```python
from build123d import *

# Parameters (mm, degrees)
EXTRUDE_1_DEPTH        = 3
SKETCH_2_R             = 4
EXTRUDE_2_DEPTH        = 10
PATTERN_LINEAR_1_COUNT = 3
PATTERN_LINEAR_1_PITCH = 20
SKETCH_3_R             = 1.5
CUT_EXTRUDE_1_DEPTH    = 65
SKETCH_4_R             = 2.5
CUT_EXTRUDE_2_DEPTH    = 66.192024052


with BuildPart() as part:
    # 草图1 → 凸台-拉伸1 (new body)
    with BuildSketch(Plane(origin=(0, 0, 0), x_dir=(1, 0, 0), z_dir=(0, 1, 0))):
        Polygon((0, 25), (60, 25), (60, -25), (0, -25), (0, -15), (5, -15), (5, -5), (0, -5), (0, 5), (5, 5), (5, 15), (0, 15), align=None)
    extrude(amount=EXTRUDE_1_DEPTH)

    # 草图2 → 凸台-拉伸2 (add)
    with BuildSketch(Plane.XY.offset(-25)):
        with Locations((0, 4)):
            Circle(SKETCH_2_R)
    extrude_2 = extrude(amount=EXTRUDE_2_DEPTH)

    # 阵列(线性)1: 凸台-拉伸2 ×3
    with Locations(*[(0, 0, i * PATTERN_LINEAR_1_PITCH) for i in range(1, PATTERN_LINEAR_1_COUNT)]):
        add(extrude_2)

    # 草图3 → 切除-拉伸1 (cut, symmetric)
    with BuildSketch(Plane.XY.offset(-25)):
        with Locations((0, 4)):
            Circle(SKETCH_3_R)
    extrude(amount=CUT_EXTRUDE_1_DEPTH, both=True, mode=Mode.SUBTRACT)

    # 草图4 → 切除-拉伸2 (cut, through all)
    with BuildSketch(Plane(origin=(0, 3, 0), x_dir=(1, 0, 0), z_dir=(0, 1, 0))):
        with Locations(Location((40, 15, 0), (0, 0, 270))):
            Circle(SKETCH_4_R)
        with Locations(Location((40, 0, 0), (0, 0, 270))):
            Circle(SKETCH_4_R)
        with Locations(Location((40, -15, 0), (0, 0, 270))):
            Circle(SKETCH_4_R)
    extrude(amount=-CUT_EXTRUDE_2_DEPTH, mode=Mode.SUBTRACT)

    # 草图10 → 切除-旋转1 (revolve, cut)
    with BuildSketch(Plane(origin=(40, 0, 0), x_dir=(0, 0, -1), z_dir=(1, 0, 0))):
        Polygon((12.5, 3), (10.5, 3), (12.5, 1), align=None)
    revolve(axis=Axis((40, 0, -15), (0, 1, 0)), mode=Mode.SUBTRACT)

    # 草图11 → 切除-旋转2 (revolve, cut)
    with BuildSketch(Plane(origin=(40, 0, 0), x_dir=(0, 0, -1), z_dir=(1, 0, 0))):
        Polygon((-2.5, 3), (-4.5, 3), (-2.5, 1), align=None)
    revolve(axis=Axis((40, 0, 0), (0, 1, 0)), mode=Mode.SUBTRACT)

    # 草图12 → 切除-旋转3 (revolve, cut)
    with BuildSketch(Plane(origin=(40, 0, 0), x_dir=(0, 0, -1), z_dir=(1, 0, 0))):
        Polygon((-17.5, 3), (-19.5, 3), (-17.5, 1), align=None)
    revolve(axis=Axis((40, 0, 15), (0, 1, 0)), mode=Mode.SUBTRACT)


solid = part.part
```
For this review, take the finished solid that the model builds, in its own axes (mm). A direction names the side the tool comes from. Coordinates: 2 decimals unless noted, no trailing zeros. Write each loop counter-clockwise with the first axis right and the second up, starting at its lowest first coordinate (ties: lowest second). Pieces come first, ordered by that corner, then holes.
(1) For pin 1 Ø1 at (x, z) = (53, -6) entering from +Y; pin 2 Ø2.5 at (x, y) = (0, 4) entering from +Z; pin 3 Ø2.5 at (y, z) = (1, -10) entering from -X; pin 4 Ø8 at (x, z) = (40, 15) entering from +Y, all flat-tipped, find the tip position at first contact; note any pin that passes through.
(2) Wall thickness on probe 1 along Y at (x, z) = (0, -21); probe 2 along Y at (x, z) = (31, -11.5); probe 3 along X at (y, z) = (1.25, -17): over which ranges is each line inside the solid? List them lowest first.
(3) Add section A-A on x = 40. Give the boundary of the cut face in (y, z).
(4) Add section C-C on z = 6.5. Give the boundary of the cut face in (x, y), then the cut area to 3 significant figures.
(5) Tool access review of faces 5 (the face through (0.806, 5.265, -19.93)), 6 (the face through (1.44, 3.17, -15)): name each direction out of +Z, -Z, +X, -X, +Y, -Y from which nothing blocks a thin tool from reaching the whole face with its end or side.
(6) Add section D-D on x = 32. Give the boundary of the cut face in (y, z), then the cut area to 3 significant figures.
(7) The part is to be moulded in two halves that separate along X. For faces 1 (the face through (5, 1, 10)), 2 (the face through (30, 0, 0)), 3 (the face through (37.56, 0.51, 14.46)), 4 (the face through (60, 1, 0)), say which applies: +X half, -X half, draft (parallel to the pull), parting line (faces both ways), or undercut.
(8) Add section B-B on y = 4. Give the boundary of the cut face in (x, z), then the cut area to 3 significant figures.
Answer sheet:
1. pin 1: stops at y = 3
1. pin 2: passes through
1. pin 3: stops at x = 5
1. pin 4: stops at y = 2.5
2. probe 1: y = 0 to 2.5, 5.5 to 8
2. probe 2: y = 0 to 3
2. probe 3: x = -2.9 to 38.11, 41.89 to 60
3. outline: (0, -25) - (3, -25) - (3, -19.5) - (1, -17.5) - (0, -17.5) - close; (0, -12.5) - (1, -12.5) - (3, -10.5) - (3, -4.5) - (1, -2.5) - (0, -2.5) - close; (0, 2.5) - (1, 2.5) - (3, 4.5) - (3, 10.5) - (1, 12.5) - (0, 12.5) - close; (0, 17.5) - (1, 17.5) - (3, 19.5) - (3, 25) - (0, 25) - close
4. outline: (5, 0) - (60, 0) - (60, 3) - (5, 3) - close
4. area: 165 mm2
5. face 5: +Z, -Z
5. face 6: -X, +Y, -Y
6. outline: (0, -25) - (3, -25) - (3, 25) - (0, 25) - close
6. area: 150 mm2
7. face 1: -X half
7. face 2: draft
7. face 3: undercut
7. face 4: +X half
8. outline: (-4, -25) - (-1.5, -25) - (-1.5, -15) - (-4, -15) - close; (-4, -5) - (-1.5, -5) - (-1.5, 5) - (-4, 5) - close; (-4, 15) - (-1.5, 15) - (-1.5, 25) - (-4, 25) - close; (1.5, -25) - (4, -25) - (4, -15) - (1.5, -15) - close; (1.5, -5) - (4, -5) - (4, 5) - (1.5, 5) - close; (1.5, 15) - (4, 15) - (4, 25) - (1.5, 25) - close
8. area: 150 mm2
